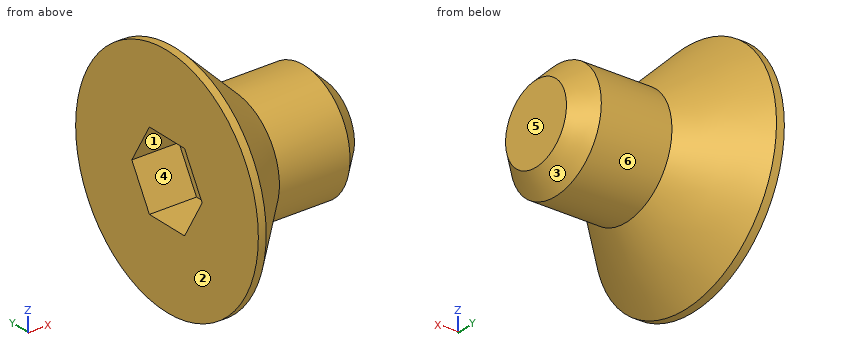
```python
from build123d import *

# Parameters (mm, degrees)
CHANFREIN1_SIZE         = 0.5
ENL_V_MAT_EXTRU_1_DEPTH = 1.2


with BuildPart() as part:
    # Esquisse1 → Révolution1 (revolve)
    with BuildSketch(Plane.XY):
        Polygon((0, 0), (0, 3), (0.2, 3), (1.7, 1.5), (4, 1.5), (4, 0), align=None)
    revolve(axis=Axis((4, 0, 0), (-1, 0, 0)))

    # Chanfrein1
    chanfrein1_edges = [part.edges().sort_by_distance(p)[0] for p in [
        (4, -1.5, 0),
    ]]
    chamfer(chanfrein1_edges, length=CHANFREIN1_SIZE)

    # Esquisse2 → Enlèv. mat.-Extru.1 (cut)
    with BuildSketch(Plane.ZY):
        Polygon((0, 1.154700538), (-1, 0.577350269), (-1, -0.577350269), (0, -1.154700538), (1, -0.577350269), (1, 0.577350269), align=None)
    extrude(amount=-ENL_V_MAT_EXTRU_1_DEPTH, mode=Mode.SUBTRACT)


solid = part.part
```
CAD build for the part. Positions are in the model's coordinates, mm. Face numbers are marked on the shaded views. A direction names the side the tool comes from. Coordinates: 2 decimals unless noted, no trailing zeros. Write each loop counter-clockwise with the first axis right and the second up, starting at its lowest first coordinate (ties: lowest second). Pieces come first, ordered by that corner, then holes.
(1) Cut at A-A, the plane x = 0.5. List the corners of the cut face in (y, z), and give its area (3 significant figures).
(2) Flat gauge pins, fed straight in: pin 1 (1.6 mm diameter, centred on y = 0.5, z = 0, fed in from -X); pin 2 (1 mm diameter, centred on x = 1, y = 1, fed in from +Z); pin 3 (1 mm diameter, centred on y = 1.5, z = -1.5, fed in from +X); pin 4 (2 mm diameter, centred on y = 0.5, z = -2, fed in from +X). Where does each tip first touch, or does it go through?
(3) Cut at C-C, the plane x = 1.1. List the corners of the cut face in (y, z), and give its area (3 significant figures).
(4) Drill centre lines: probe 1 along Z at (x, y) = (0.8, -0.2); probe 2 along X at (y, z) = (0, -0.2); probe 3 along Y at (x, z) = (1.1, 0.75). Where is each one in solid material? Low to high.
(5) Cut at B-B, the plane y = 0. List the corners of the cut face in (x, z).
(6) 3-axis set-ups, long thin cutter, end or side, ignore diameter. For the marked faces 4, 5 and 6: which of +Z, -Z, +X, -X, +Y, -Y reach the whole face in a straight line?
(7) Cut at D-D, the plane x = 2.5. List the corners of the cut face in (y, z).
(8) Two-plate mould, pull along Y, no slides. Class the marked faces 1, 2 and 3: +Y half, -Y half, draft (parallel to the pull), parting line (faces both ways), or undercut.
Geometry says:
1. outline: circle Ø5.4 at (0, 0); hole (-1.15, 0) - (-0.58, -1) - (0.58, -1) - (1.15, 0) - (0.58, 1) - (-0.58, 1) - close
1. area: 19.4 mm2
2. pin 1: stops at x = 0
2. pin 2: stops at z = 2.54
2. pin 3: stops at x = 1.58
2. pin 4: stops at x = 3.94
3. outline: circle Ø4.2 at (0, 0); hole (-1.15, 0) - (-0.58, -1) - (0.58, -1) - (1.15, 0) - (0.58, 1) - (-0.58, 1) - close
3. area: 10.4 mm2
4. probe 1: z = -2.39 to -1, 1 to 2.39
4. probe 2: x = 1.2 to 4
4. probe 3: y = -1.96 to -0.72, 0.72 to 1.96
5. outline: (0, -3) - (0.2, -3) - (1.7, -1.5) - (3.5, -1.5) - (4, -1) - (4, 1) - (3.5, 1.5) - (1.7, 1.5) - (0.2, 3) - (0, 3) - (0, 1) - (1.2, 1) - (1.2, -1) - (0, -1) - close
6. face 4: -X
6. face 5: +Z, -Z, +X, +Y, -Y
6. face 6: +X
7. outline: circle Ø3 at (0, 0)
8. face 1: undercut
8. face 2: draft
8. face 3: parting line
